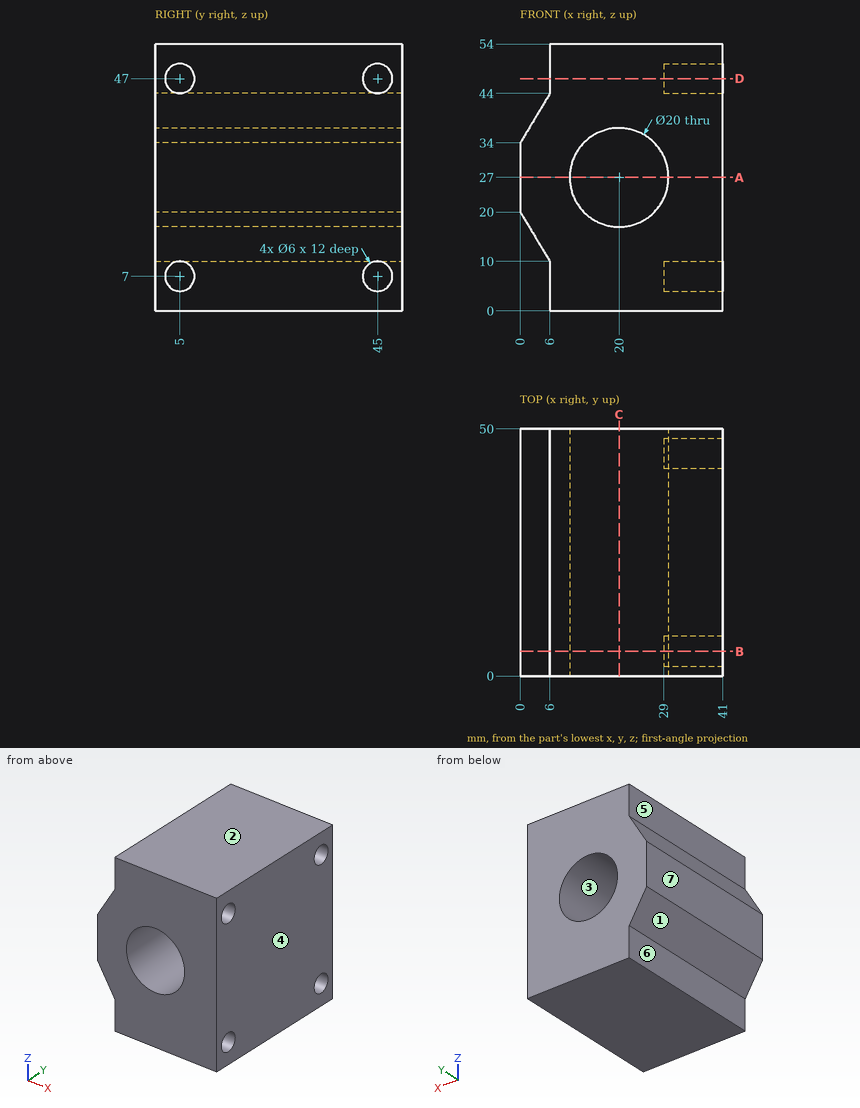
Input: dimensioned drawing with shaded views. Units: mm. Origin: part minimum x, y, z. A direction names the side the tool comes from. Give positions to 0.01 mm unless a question says otherwise; leave off trailing zeros. Write each loop counter-clockwise with the first axis right and the second up, starting at its lowest first coordinate (ties: lowest second). Pieces come first, ordered by that corner, then holes. Notation, with made-up numbers: M -1,7.25 L 17,7.25 A32 ccw 17,33.25 Z; hole C 52,10.5 d7. An arc over 180 degrees is marked long. Write item = value, one per line. Start each with the question number.
1) Material intervals for line 1 along Z through (x, y) = (36.25, 45); line 2 along X through (y, z) = (27, 3.5); line 3 along Z through (x, y) = (13, 19.5), sorted ascending. Write a range as [from, to].
2) Cut plane B-B on y = 5. Return the cut outline in (x, z).
3) Cut plane D-D on z = 47. Return the cut outline in (x, y), then the cut area to 3 significant figures.
4) Cut plane A-A on z = 27. Return the cut outline in (x, y), then the cut area to 3 significant figures.
5) Reachability of the marked faces 5, 6 and 7 from +Z, -Z, +X, -X, +Y, -Y: full face, straight path, thin tool, end or side. Return the list, or none.
6) Cut plane C-C on x = 20. Return the cut outline in (y, z), then the cut area to 3 significant figures.
7) Draft query along Z for the marked faces 1, 2, 3 and 4. Return one class per face: +Z half, -Z half, draft (parallel to the pull), parting line (faces both ways), or undercut.
8) First-contact query: pin 1 Ø3 at (y, z) = (19, 37) entering from -X; pin 2 Ø3 at (y, z) = (45, 6.5) entering from +X; pin 3 Ø9.5 at (y, z) = (45, 47) entering from -X; pin 4 Ø16 at (x, z) = (20, 27) entering from +Y. Flat tips, straight axial feed; report the tip coordinate or a pass-through.
Solved:
q1.line_1 = [0, 4], [10, 44], [50, 54]
q1.line_2 = [6, 41]
q1.line_3 = [0, 19.86], [34.14, 54]
q2.outline = M 0,20 L 6,10 L 6,0 L 41,0 L 41,4 L 29,4 L 29,10 L 41,10 L 41,44 L 29,44 L 29,50 L 41,50 L 41,54 L 6,54 L 6,44 L 0,34 Z; hole C 20,27 d20
q3.outline = M 6,0 L 41,0 L 41,2 L 29,2 L 29,8 L 41,8 L 41,42 L 29,42 L 29,48 L 41,48 L 41,50 L 6,50 Z
q3.area = 1,610 mm2
q4.outline = M 0,0 L 10,0 L 10,50 L 0,50 Z; M 30,0 L 41,0 L 41,50 L 30,50 Z
q4.area = 1,050 mm2
q5.face_5 = +Z, -X, +Y, -Y
q5.face_6 = -Z, -X, +Y, -Y
q5.face_7 = +Z, -Z, -X, +Y, -Y
q6.outline = M 0,0 L 50,0 L 50,17 L 0,17 Z; M 0,37 L 50,37 L 50,54 L 0,54 Z
q6.area = 1,700 mm2
q7.face_1 = -Z half
q7.face_2 = +Z half
q7.face_3 = undercut
q7.face_4 = draft
q8.pin_1 = 0.9
q8.pin_2 = 29
q8.pin_3 = 4.95
q8.pin_4 = through
